Work out the finished part from the listing and answer in its coordinate system (mm). A direction names the side the tool comes from. Round coordinates to 2 decimals unless told otherwise and drop trailing zeros. Write each loop counter-clockwise with the first axis right and the second up, starting at its lowest first coordinate (ties: lowest second). Pieces come first, ordered by that corner, then holes.
1. Find section B-B (y = 9). Write down the section's boundary in (x, z).
2. Flat-ended cylindrical pins translate along their axes: pin 1 Ø5 at (x, y) = (-52.5, -30.5) entering from +Z; pin 2 Ø5.5 at (x, y) = (-83, -35) entering from +Z; pin 3 Ø5.5 at (x, y) = (-83, 35) entering from -Z. Find the tip coordinate at first contact, or state that the pin passes through.
3. Find section A-A (x = 16). Write down the section's boundary in (y, z), and give its area (3 significant figures).
4. Determine the mould class of faces 1 (the face through (0, 39, 15)), 2 (the face through (76, 27, 9)) for opening direction X: pulls with the +X half, pulls with the -X half, needs draft (parallel to the pull), parting line crosses it, or undercut.
5. Straight lines are drawn through the part: probe 1 along Y at (x, z) = (83, 1.9); probe 2 along Y at (x, z) = (-66.5, 7.25); probe 3 along X at (y, z) = (10.5, 5.75). For each, find the intervals that lie inside material, in ascending order.
6. A tool of negligible diameter and unlimited length cuts with its end or side. For faces 3 (the face through (83.521, 38.966, 1.282)), 4 (the face through (81.415, 36.453, 8.887)), 5 (the face through (-78, 29, 9)), from which of +Z, -Z, +X, -X, +Y, -Y can it reach the whole face along a straight path? Write none if from no direction.
7. Find section C-C (z = 11). Count the separate pieces of the cut face and the enclosed holes in it, and give its area (3 significant figures).
```python
from build123d import *

# Parameters (mm, degrees)
SKETCH1_W                                   = 176
SKETCH1_H                                   = 80
BOSS_EXTRUDE1_DEPTH                         = 38.5
SKETCH2_W                                   = 168
SKETCH2_H                                   = 72
CUT_EXTRUDE1_DEPTH                          = 35
FILLET2_R                                   = 5
SKETCH8_W                                   = 8
SKETCH8_H                                   = 20
SKETCH8_H_2                                 = 8
BOSS_EXTRUDE2_DEPTH                         = 35
FILLET4_R                                   = 3
FILLET5_R                                   = 5
M4_TAPPED_HOLE1_D                           = 3.3
M4_TAPPED_HOLE1_DEPTH                       = 11.5
M4_TAPPED_HOLE1_TIP                         = 0.991420021
BOSS_EXTRUDE3_START                         = 1.5
BOSS_EXTRUDE3_DEPTH                         = 1.5
SKETCH25_W                                  = 192.92581759
SKETCH25_H                                  = 92.850065769
CUT_EXTRUDE4_DEPTH                          = 25
CBORE_FOR_M4_CHEESE_HEAD_SCREW2_D           = 4.3
CBORE_FOR_M4_CHEESE_HEAD_SCREW2_CBORE_D     = 8
CBORE_FOR_M4_CHEESE_HEAD_SCREW2_CBORE_DEPTH = 2.6


with BuildPart() as part:
    # Sketch1 → Boss-Extrude1 (new body)
    with BuildSketch(Plane.XY):
        Rectangle(SKETCH1_W, SKETCH1_H)
    extrude(amount=BOSS_EXTRUDE1_DEPTH)

    # Sketch2 → Cut-Extrude1 (cut)
    with BuildSketch(Plane.XY.offset(38.5)):
        Rectangle(SKETCH2_W, SKETCH2_H)
    extrude(amount=-CUT_EXTRUDE1_DEPTH, mode=Mode.SUBTRACT)

    # Fillet2
    fillet2_edges = [part.edges().sort_by_distance(p)[0] for p in [
        (-88, 40, 19.25),
        (88, 40, 19.25),
        (88, -40, 19.25),
        (-88, -40, 19.25),
    ]]
    fillet(fillet2_edges, radius=FILLET2_R)

    # Sketch8 → Boss-Extrude2 (add)
    with BuildSketch(Plane.XY.offset(3.5)):
        with Locations((80, 26)):
            Rectangle(SKETCH8_W, SKETCH8_H)
        with Locations((80, -32)):
            Rectangle(SKETCH8_W, SKETCH8_H_2)
        with Locations((-80, -26)):
            Rectangle(SKETCH8_W, SKETCH8_H)
        with Locations((-80, 32)):
            Rectangle(SKETCH8_W, SKETCH8_H_2)
    extrude(amount=BOSS_EXTRUDE2_DEPTH)

    # Fillet4
    fillet4_edges = [part.edges().sort_by_distance(p)[0] for p in [
        (76, 36, 21),
        (84, 16, 21),
        (84, -28, 21),
        (76, -36, 21),
        (-76, -36, 21),
        (-84, -16, 21),
        (-84, 28, 21),
        (-76, 36, 21),
    ]]
    fillet(fillet4_edges, radius=FILLET4_R)

    # Fillet5
    fillet5_edges = [part.edges().sort_by_distance(p)[0] for p in [
        (-76, -16, 21),
        (76, -28, 21),
        (76, 16, 21),
        (-76, 28, 21),
    ]]
    fillet(fillet5_edges, radius=FILLET5_R - 0.0001)  # a hair under: the kernel refuses the full size

    # M4 Tapped Hole1
    with Locations(Plane.XY.offset(38.5)):
        with Locations((-83, -35), (83, 35), (-83, 35), (83, -35)):
            Hole(M4_TAPPED_HOLE1_D / 2, depth=M4_TAPPED_HOLE1_DEPTH)
            with Locations((0, 0, -(M4_TAPPED_HOLE1_DEPTH + M4_TAPPED_HOLE1_TIP / 2))):  # 118° drill point
                Cone(0, M4_TAPPED_HOLE1_D / 2, M4_TAPPED_HOLE1_TIP, mode=Mode.SUBTRACT)

    # Sketch9 → Boss-Extrude3 (add)
    with BuildSketch(Plane.XY.offset(38.5).offset(BOSS_EXTRUDE3_START)):
        with BuildLine():
            Line((73, 37.5), (-73, 37.5))
            ThreePointArc((-73, 37.5), (-76.181980515, 36.181980515), (-77.5, 33))
            ThreePointArc((-77.5, 33), (-78.525126266, 30.525126266), (-81, 29.5))
            ThreePointArc((-81, 29.5), (-84.181980515, 28.181980515), (-85.5, 25))
            Line((-85.5, 25), (-85.5, -13))
            ThreePointArc((-85.5, -13), (-84.181980515, -16.181980515), (-81, -17.5))
            ThreePointArc((-81, -17.5), (-78.525126266, -18.525126266), (-77.5, -21))
            Line((-77.5, -21), (-77.5, -33))
            ThreePointArc((-77.5, -33), (-76.181980515, -36.181980515), (-73, -37.5))
            Line((-73, -37.5), (73, -37.5))
            ThreePointArc((73, -37.5), (76.181980515, -36.181980515), (77.5, -33))
            ThreePointArc((77.5, -33), (78.525126266, -30.525126266), (81, -29.5))
            ThreePointArc((81, -29.5), (84.181980515, -28.181980515), (85.5, -25))
            Line((85.5, -25), (85.5, 13))
            ThreePointArc((85.5, 13), (84.181980515, 16.181980515), (81, 17.5))
            ThreePointArc((81, 17.5), (78.525126266, 18.525126266), (77.5, 21))
            Line((77.5, 21), (77.5, 33))
            ThreePointArc((77.5, 33), (76.181980515, 36.181980515), (73, 37.5))
        make_face()
        with BuildLine():
            Line((73, 36), (-73, 36))
            ThreePointArc((-73, 36), (-75.121320344, 35.121320344), (-76, 33))
            ThreePointArc((-76, 33), (-77.464466094, 29.464466094), (-81, 28))
            ThreePointArc((-81, 28), (-83.121320344, 27.121320344), (-84, 25))
            Line((-84, 25), (-84, -13))
            ThreePointArc((-84, -13), (-83.121320344, -15.121320344), (-81, -16))
            ThreePointArc((-81, -16), (-77.464466094, -17.464466094), (-76, -21))
            Line((-76, -21), (-76, -33))
            ThreePointArc((-76, -33), (-75.121320344, -35.121320344), (-73, -36))
            Line((-73, -36), (73, -36))
            ThreePointArc((73, -36), (75.121320344, -35.121320344), (76, -33))
            ThreePointArc((76, -33), (77.464466094, -29.464466094), (81, -28))
            ThreePointArc((81, -28), (83.121320344, -27.121320344), (84, -25))
            Line((84, -25), (84, 13))
            ThreePointArc((84, 13), (83.121320344, 15.121320344), (81, 16))
            ThreePointArc((81, 16), (77.464466094, 17.464466094), (76, 21))
            Line((76, 21), (76, 33))
            ThreePointArc((76, 33), (75.121320344, 35.121320344), (73, 36))
        make_face(mode=Mode.SUBTRACT)
    extrude(amount=-BOSS_EXTRUDE3_DEPTH)

    # Sketch25 → Cut-Extrude4 (cut)
    with BuildSketch(Plane.XY.offset(40)):
        with Locations((-2.348347967, 1.083852907)):
            Rectangle(SKETCH25_W, SKETCH25_H)
    extrude(amount=-CUT_EXTRUDE4_DEPTH, mode=Mode.SUBTRACT)

    # CBORE for M4 Cheese Head Screw2 (through all)
    with Locations(Plane(origin=(0, 0, 0), x_dir=(-1, 0, 0), z_dir=(0, 0, -1))):
        with Locations((-83, 35), (83, 35), (83, -35), (-83, -35)):
            CounterBoreHole(CBORE_FOR_M4_CHEESE_HEAD_SCREW2_D / 2, CBORE_FOR_M4_CHEESE_HEAD_SCREW2_CBORE_D / 2, CBORE_FOR_M4_CHEESE_HEAD_SCREW2_CBORE_DEPTH)


solid = part.part
```
Worked answers:
1. outline: (-88, 0) - (88, 0) - (88, 15) - (84, 15) - (84, 3.5) - (-84, 3.5) - (-84, 15) - (-88, 15) - close
2. pin 1: stops at z = 3.5
2. pin 2: stops at z = 15
2. pin 3: stops at z = 2.6
3. outline: (-40, 0) - (40, 0) - (40, 15) - (36, 15) - (36, 3.5) - (-36, 3.5) - (-36, 15) - (-40, 15) - close
3. area: 372 mm2
4. face 1: needs draft
4. face 2: undercut
5. probe 1: y = -40 to -39, -31 to 31, 39 to 40
5. probe 2: y = -40 to -36, 36 to 40
5. probe 3: x = -88 to -84, 84 to 88
6. face 3: -Z
6. face 4: +Z, -Z
6. face 5: +Z
7. separate pieces: 1
7. enclosed holes: 5
7. area: 2,350 mm2
